```python
from build123d import *

# Parameters (mm, degrees)
F0_W     = 50.8
F0_H     = 38.1
F0_W_2   = 1.3446661346
F0_H_2   = 9.9171942893
F1_DEPTH = 12.7
F2_DEPTH = 25.4


with BuildPart() as f1:
    # F0 (on Front) → F1 (new body, symmetric)
    with BuildSketch(Plane.XZ):
        with Locations((-36.0804582015, 47.4701705396)):
            Rectangle(F0_W, F0_H)
        with BuildLine():
            add(Edge.make_bspline(
                [(-56.1243173839, 44.267506293), (-56.9058904973, 43.4397595518), (-58.2640708644, 43.4397595518)],
                knots=[0, 0, 0, 1, 1, 1], degree=2))
            add(Edge.make_bspline(
                [(-58.2640708644, 43.4397595518), (-60.7844752273, 43.4397595518), (-61.255220993, 46.0457540539)],
                knots=[0, 0, 0, 1, 1, 1], degree=2))
            Line((-61.255220993, 46.0457540539), (-59.9398356955, 46.2642341461))
            add(Edge.make_bspline(
                [(-59.9398356955, 46.2642341461), (-59.8114504867, 45.4466230794), (-59.368859372, 44.9893915462)],
                knots=[0, 0, 0, 1, 1, 1], degree=2))
            add(Edge.make_bspline(
                [(-59.368859372, 44.9893915462), (-58.9262682573, 44.5321600129), (-58.2573137482, 44.5321600129)],
                knots=[0, 0, 0, 1, 1, 1], degree=2))
            add(Edge.make_bspline(
                [(-58.2573137482, 44.5321600129), (-57.5252928206, 44.5321600129), (-57.1029730547, 45.0355651739)],
                knots=[0, 0, 0, 1, 1, 1], degree=2))
            add(Edge.make_bspline(
                [(-57.1029730547, 45.0355651739), (-56.6806532888, 45.5389703348), (-56.6806532888, 46.5097427034)],
                knots=[0, 0, 0, 1, 1, 1], degree=2))
            Line((-56.6806532888, 46.5097427034), (-56.6806532888, 52.4019480771))
            Line((-56.6806532888, 52.4019480771), (-58.5884124446, 52.4019480771))
            Line((-58.5884124446, 52.4019480771), (-58.5884124446, 53.4988532824))
            Line((-58.5884124446, 53.4988532824), (-55.3427442705, 53.4988532824))
            Line((-55.3427442705, 53.4988532824), (-55.3427442705, 46.5390235405))
            add(Edge.make_bspline(
                [(-55.3427442705, 46.5390235405), (-55.3427442705, 45.0952530341), (-56.1243173839, 44.267506293)],
                knots=[0, 0, 0, 1, 1, 1], degree=2))
        make_face(mode=Mode.SUBTRACT)
        Polygon((-44.6867719374, 43.5816589932), (-46.058466537, 43.5816589932), (-47.1914096957, 46.4827142384), (-51.7096680977, 46.4827142384), (-52.8516207447, 43.5816589932), (-54.2435866931, 43.5816589932), (-50.1983264288, 53.4988532824), (-48.6689657833, 53.4988532824), align=None, mode=Mode.SUBTRACT)
        Polygon((-35.1051810888, 53.4988532824), (-39.1526937251, 43.5816589932), (-40.5469120456, 43.5816589932), (-44.5944246819, 53.4988532824), (-43.1799350127, 53.4988532824), (-40.4342934413, 46.5164998196), (-39.841919583, 44.7641543377), (-39.2517980968, 46.5164998196), (-36.519670758, 53.4988532824), align=None, mode=Mode.SUBTRACT)
        with Locations((-33.038629701, 48.5402561378)):
            Rectangle(F0_W_2, F0_H_2, mode=Mode.SUBTRACT)
        Polygon((-22.0414229971, 43.5816589932), (-29.8549017592, 43.5816589932), (-29.8549017592, 53.4988532824), (-22.3297266239, 53.4988532824), (-22.3297266239, 52.4019480771), (-28.5102356245, 52.4019480771), (-28.5102356245, 49.2193463214), (-22.7531725759, 49.2193463214), (-22.7531725759, 48.1359553486), (-28.5102356245, 48.1359553486), (-28.5102356245, 44.6808165705), (-22.0414229971, 44.6808165705), align=None, mode=Mode.SUBTRACT)
        with BuildLine():
            Line((-11.6805114071, 43.5816589932), (-13.2278910293, 43.5816589932))
            Line((-13.2278910293, 43.5816589932), (-15.8046046943, 47.6989951641))
            Line((-15.8046046943, 47.6989951641), (-18.8948591946, 47.6989951641))
            Line((-18.8948591946, 47.6989951641), (-18.8948591946, 43.5816589932))
            Line((-18.8948591946, 43.5816589932), (-20.2395253293, 43.5816589932))
            Line((-20.2395253293, 43.5816589932), (-20.2395253293, 53.4988532824))
            Line((-20.2395253293, 53.4988532824), (-15.5726103696, 53.4988532824))
            add(Edge.make_bspline(
                [(-15.5726103696, 53.4988532824), (-13.8968455385, 53.4988532824), (-12.9857610302, 52.7499395642)],
                knots=[0, 0, 0, 1, 1, 1], degree=2))
            add(Edge.make_bspline(
                [(-12.9857610302, 52.7499395642), (-12.0746765219, 52.0010258461), (-12.0746765219, 50.6631168277)],
                knots=[0, 0, 0, 1, 1, 1], degree=2))
            add(Edge.make_bspline(
                [(-12.0746765219, 50.6631168277), (-12.0746765219, 49.5572021341), (-12.7188549382, 48.8037836717)],
                knots=[0, 0, 0, 1, 1, 1], degree=2))
            add(Edge.make_bspline(
                [(-12.7188549382, 48.8037836717), (-13.3630333544, 48.0503652094), (-14.4959765131, 47.854408838)],
                knots=[0, 0, 0, 1, 1, 1], degree=2))
            Line((-14.4959765131, 47.854408838), (-11.6805114071, 43.5816589932))
        make_face(mode=Mode.SUBTRACT)
    extrude(amount=F1_DEPTH, both=True)

    # F0 (on Front) → F2 (join)
    with BuildSketch(Plane.XZ):
        with Locations((-36.0804582015, 47.4701705396)):
            Rectangle(F0_W, F0_H)
        with BuildLine():
            add(Edge.make_bspline(
                [(-56.1243173839, 44.267506293), (-56.9058904973, 43.4397595518), (-58.2640708644, 43.4397595518)],
                knots=[0, 0, 0, 1, 1, 1], degree=2))
            add(Edge.make_bspline(
                [(-58.2640708644, 43.4397595518), (-60.7844752273, 43.4397595518), (-61.255220993, 46.0457540539)],
                knots=[0, 0, 0, 1, 1, 1], degree=2))
            Line((-61.255220993, 46.0457540539), (-59.9398356955, 46.2642341461))
            add(Edge.make_bspline(
                [(-59.9398356955, 46.2642341461), (-59.8114504867, 45.4466230794), (-59.368859372, 44.9893915462)],
                knots=[0, 0, 0, 1, 1, 1], degree=2))
            add(Edge.make_bspline(
                [(-59.368859372, 44.9893915462), (-58.9262682573, 44.5321600129), (-58.2573137482, 44.5321600129)],
                knots=[0, 0, 0, 1, 1, 1], degree=2))
            add(Edge.make_bspline(
                [(-58.2573137482, 44.5321600129), (-57.5252928206, 44.5321600129), (-57.1029730547, 45.0355651739)],
                knots=[0, 0, 0, 1, 1, 1], degree=2))
            add(Edge.make_bspline(
                [(-57.1029730547, 45.0355651739), (-56.6806532888, 45.5389703348), (-56.6806532888, 46.5097427034)],
                knots=[0, 0, 0, 1, 1, 1], degree=2))
            Line((-56.6806532888, 46.5097427034), (-56.6806532888, 52.4019480771))
            Line((-56.6806532888, 52.4019480771), (-58.5884124446, 52.4019480771))
            Line((-58.5884124446, 52.4019480771), (-58.5884124446, 53.4988532824))
            Line((-58.5884124446, 53.4988532824), (-55.3427442705, 53.4988532824))
            Line((-55.3427442705, 53.4988532824), (-55.3427442705, 46.5390235405))
            add(Edge.make_bspline(
                [(-55.3427442705, 46.5390235405), (-55.3427442705, 45.0952530341), (-56.1243173839, 44.267506293)],
                knots=[0, 0, 0, 1, 1, 1], degree=2))
        make_face(mode=Mode.SUBTRACT)
        Polygon((-44.6867719374, 43.5816589932), (-46.058466537, 43.5816589932), (-47.1914096957, 46.4827142384), (-51.7096680977, 46.4827142384), (-52.8516207447, 43.5816589932), (-54.2435866931, 43.5816589932), (-50.1983264288, 53.4988532824), (-48.6689657833, 53.4988532824), align=None, mode=Mode.SUBTRACT)
        Polygon((-35.1051810888, 53.4988532824), (-39.1526937251, 43.5816589932), (-40.5469120456, 43.5816589932), (-44.5944246819, 53.4988532824), (-43.1799350127, 53.4988532824), (-40.4342934413, 46.5164998196), (-39.841919583, 44.7641543377), (-39.2517980968, 46.5164998196), (-36.519670758, 53.4988532824), align=None, mode=Mode.SUBTRACT)
        with Locations((-33.038629701, 48.5402561378)):
            Rectangle(F0_W_2, F0_H_2, mode=Mode.SUBTRACT)
        Polygon((-22.0414229971, 43.5816589932), (-29.8549017592, 43.5816589932), (-29.8549017592, 53.4988532824), (-22.3297266239, 53.4988532824), (-22.3297266239, 52.4019480771), (-28.5102356245, 52.4019480771), (-28.5102356245, 49.2193463214), (-22.7531725759, 49.2193463214), (-22.7531725759, 48.1359553486), (-28.5102356245, 48.1359553486), (-28.5102356245, 44.6808165705), (-22.0414229971, 44.6808165705), align=None, mode=Mode.SUBTRACT)
        with BuildLine():
            Line((-11.6805114071, 43.5816589932), (-13.2278910293, 43.5816589932))
            Line((-13.2278910293, 43.5816589932), (-15.8046046943, 47.6989951641))
            Line((-15.8046046943, 47.6989951641), (-18.8948591946, 47.6989951641))
            Line((-18.8948591946, 47.6989951641), (-18.8948591946, 43.5816589932))
            Line((-18.8948591946, 43.5816589932), (-20.2395253293, 43.5816589932))
            Line((-20.2395253293, 43.5816589932), (-20.2395253293, 53.4988532824))
            Line((-20.2395253293, 53.4988532824), (-15.5726103696, 53.4988532824))
            add(Edge.make_bspline(
                [(-15.5726103696, 53.4988532824), (-13.8968455385, 53.4988532824), (-12.9857610302, 52.7499395642)],
                knots=[0, 0, 0, 1, 1, 1], degree=2))
            add(Edge.make_bspline(
                [(-12.9857610302, 52.7499395642), (-12.0746765219, 52.0010258461), (-12.0746765219, 50.6631168277)],
                knots=[0, 0, 0, 1, 1, 1], degree=2))
            add(Edge.make_bspline(
                [(-12.0746765219, 50.6631168277), (-12.0746765219, 49.5572021341), (-12.7188549382, 48.8037836717)],
                knots=[0, 0, 0, 1, 1, 1], degree=2))
            add(Edge.make_bspline(
                [(-12.7188549382, 48.8037836717), (-13.3630333544, 48.0503652094), (-14.4959765131, 47.854408838)],
                knots=[0, 0, 0, 1, 1, 1], degree=2))
            Line((-14.4959765131, 47.854408838), (-11.6805114071, 43.5816589932))
        make_face(mode=Mode.SUBTRACT)
    extrude(amount=F2_DEPTH)


solid = f1.part
```
Work out the finished part from the listing and answer in its coordinate system (mm). A direction names the side the tool comes from. Coordinates: 2 decimals unless noted, no trailing zeros. Loops run counter-clockwise (first coordinate to the right, second up) from the corner with the lowest first, then second, coordinate; pieces in that order, holes last. Notation, with made-up numbers: (45, 82.25) - (98, 82.25) arc R25 cw to (98, 119.25) - close; hole circle Ø2 at (27, -5.5). An arc over 180 degrees is marked (long way). Use a Markdown table: item, result.
Item 1: The mould has two halves that part along Z. Classify faces 3 (the flat face through (-36, 12.7, 48)), 4 (the flat face through (-37.1, -6.08, 48.61)), 5 (the flat face through (-36, -7, 66.52)): +Z half, -Z half, draft (parallel to the pull), parting line (faces both ways), or undercut.
Evaluation:
| item | result |
|---|---|
| face 3 | draft |
| face 4 | undercut |
| face 5 | +Z half |
Item 2: Find section C-C, the plane x = -38. Determine the outline of the cut face in (y, z), and give its area (3 significant figures).
Evaluation:
| item | result |
|---|---|
| outline | (-25.4, 28.42) - (12.7, 28.42) - (12.7, 46.41) - (-25.4, 46.41) - close; (-25.4, 49.72) - (12.7, 49.72) - (12.7, 66.52) - (-25.4, 66.52) - close |
| area | 1,330 mm2 |
Item 3: For faces 1 (the flat face through (-10.68, -7, 47)), 2 (the flat face through (-28.51, -6, 51)), determine the directions among +Z, -Z, +X, -X, +Y, -Y from which every point of the face is accessible in a straight line to the end or side of a thin tool.
Evaluation:
| item | result |
|---|---|
| face 1 | +Z, -Z, +X, +Y, -Y |
| face 2 | +Y, -Y |
Item 4: Find section B-B, the plane y = 10. State how many separate pieces and enclosed holes the cut face has, and give its area (3 significant figures).
Evaluation:
| item | result |
|---|---|
| separate pieces | 1 |
| enclosed holes | 6 |
| area | 1,750 mm2 |
Item 5: Find section A-A, the plane x = -51. Determine the outline of the cut face in (y, z).
Evaluation:
| item | result |
|---|---|
| outline | (-25.4, 28.42) - (12.7, 28.42) - (12.7, 46.48) - (-25.4, 46.48) - close; (-25.4, 51.53) - (12.7, 51.53) - (12.7, 66.52) - (-25.4, 66.52) - close |
Item 6: Consider probe 1 along Z at (x, y) = (-24.5, -14.5); probe 2 along Z at (x, y) = (-13.5, -8); probe 3 along Z at (x, y) = (-50, -7.5). Determine where each line is inside the solid, lowest interval first. Write a range as from..to.
Evaluation:
| item | result |
|---|---|
| probe 1 | z = 28.42..43.58, 44.68..48.14, 49.22..52.4, 53.5..66.52 |
| probe 2 | z = 28.42..44.02, 46.34..48.18, 53.08..66.52 |
| probe 3 | z = 28.42..46.48, 53.5..66.52 |
